```python
from build123d import *

# Parameters (mm, degrees)
SKETCH1_W           = 333
SKETCH1_H           = 544
SKETCH1_W_2         = 48
SKETCH1_H_2         = 6
SKETCH1_W_3         = 69
SKETCH1_W_4         = 6
SKETCH1_H_3         = 20
SKETCH1_W_5         = 20
BOSS_EXTRUDE1_DEPTH = 6
SKETCH2_W           = 143.5
SKETCH2_H           = 290
CUT_EXTRUDE1_DEPTH  = 6


with BuildPart() as part:
    # Sketch1 → Boss-Extrude1 (new body)
    with BuildSketch(Plane.XY):
        with Locations((27.644903204, -172)):
            Rectangle(SKETCH1_W, SKETCH1_H)
        with Locations((139.644903204, 47)):
            Rectangle(SKETCH1_W_2, SKETCH1_H_2, mode=Mode.SUBTRACT)
        with Locations((139.644903204, 77)):
            Rectangle(SKETCH1_W_3, SKETCH1_H_2, mode=Mode.SUBTRACT)
        with Locations((139.644903204, -101)):
            Rectangle(SKETCH1_W_2, SKETCH1_H_2, mode=Mode.SUBTRACT)
        with Locations((139.644903204, -131)):
            Rectangle(SKETCH1_W_3, SKETCH1_H_2, mode=Mode.SUBTRACT)
        with Locations((-84.355096796, 77)):
            Rectangle(SKETCH1_W_3, SKETCH1_H_2, mode=Mode.SUBTRACT)
        with Locations((-84.355096796, 47)):
            Rectangle(SKETCH1_W_2, SKETCH1_H_2, mode=Mode.SUBTRACT)
        with Locations((-84.355096796, -101)):
            Rectangle(SKETCH1_W_2, SKETCH1_H_2, mode=Mode.SUBTRACT)
        with Locations((-84.355096796, -131)):
            Rectangle(SKETCH1_W_3, SKETCH1_H_2, mode=Mode.SUBTRACT)
        with Locations((27.644903204, -394)):
            Rectangle(SKETCH1_W_4, SKETCH1_H_3, mode=Mode.SUBTRACT)
        with Locations((27.644903204, -334)):
            Rectangle(SKETCH1_W_4, SKETCH1_H_3, mode=Mode.SUBTRACT)
        with Locations((-62.855096796, -431)):
            Rectangle(SKETCH1_W_5, SKETCH1_H_2, mode=Mode.SUBTRACT)
        with Locations((-122.855096796, -431)):
            Rectangle(SKETCH1_W_5, SKETCH1_H_2, mode=Mode.SUBTRACT)
    extrude(amount=BOSS_EXTRUDE1_DEPTH)

    # Sketch2 → Cut-Extrude1 (cut)
    with BuildSketch(Plane.XY.offset(6)):
        with Locations((122.394903204, -299)):
            Rectangle(SKETCH2_W, SKETCH2_H)
    extrude(amount=-CUT_EXTRUDE1_DEPTH, mode=Mode.SUBTRACT)


solid = part.part
```
Input: part model. Units: mm. Frame: model coordinates. Give positions to 0.01 mm unless a question says otherwise; leave off trailing zeros. Write each loop counter-clockwise with the first axis right and the second up, starting at its lowest first coordinate (ties: lowest second). Pieces come first, ordered by that corner, then holes. Notation, with made-up numbers: (26.5, 26) - (48.5, 26) arc R9 ccw to (48.5, 30) - close; hole circle Ø2 at (87, 9). An arc over 180 degrees is marked (long way). Write item = value, one per line. Start each with the question number.
1) Cut plane A-A (x = 77.5). Return loops of the section in (y, z), and give its area (3 significant figures).
2) Pin query (flat end, axial travel): pin 1 (1.8 mm diameter, centred on y = -335, z = 3.5, fed in from +X). Return the tip coordinate at first contact, or that it passes through.
3) Cut plane C-C (y = -361). Return loops of the section in (x, z).
4) Cut plane B-B (z = 4.5). Give the number of separate pieces and of enclosed holes in the cut face, and give its area (3 significant figures).
5) Material intervals for L1, parallel to Y at x = -107.5, z = 3.55; L2, parallel to Y at x = -113, z = 4.25; L3, parallel to X at y = -402, z = 4.75, sorted ascending. Write a range as [from, to].
Answers follow:
q1.outline = (-154, 0) - (100, 0) - (100, 6) - (-154, 6) - close
q1.area = 1,520 mm^2
q2.pin_1 = 50.64
q3.outline = (-138.86, 0) - (50.64, 0) - (50.64, 6) - (-138.86, 6) - close
q4.separate_pieces = 1
q4.enclosed_holes = 12
q4.area = 136,000 mm^2
q5.L1 = [-444, -134], [-128, -104], [-98, 44], [50, 74], [80, 100]
q5.L2 = [-444, -434], [-428, -134], [-128, 74], [80, 100]
q5.L3 = [-138.86, 24.64], [30.64, 50.64]
